from build123d import *

# Parameters (mm, degrees)
BOSS_EXTRUDE1_DEPTH = 6
SKETCH3_W           = 96
SKETCH3_H           = 45.5
BOSS_EXTRUDE2_DEPTH = 6
CUT_EXTRUDE1_DEPTH  = 6
CUT_EXTRUDE2_DEPTH  = 91.403621508
SKETCH9_W           = 27
SKETCH9_H           = 33.5
CUT_EXTRUDE3_DEPTH  = 91.403621508
CHAMFER1_SIZE       = 2
SKETCH11_R          = 2
CUT_EXTRUDE4_DEPTH  = 91.403621508
CUT_EXTRUDE6_START  = 0.01
SKETCH12_W          = 8
SKETCH12_H          = 6.6
CUT_EXTRUDE6_DEPTH  = 91.493120288


with BuildPart() as part:
    # Sketch2 → Boss-Extrude1 (new body)
    with BuildSketch(Plane(origin=(0, 0, 0), x_dir=(1, 0, 0), z_dir=(0, 1, 0))):
        with BuildLine():
            Line((27.190997647, 15.698729811), (53.17175976, 30.698729811))
            Line((53.17175976, 30.698729811), (48, 39.65648048))
            Line((48, 39.65648048), (48, 50))
            Line((48, 50), (-48, 50))
            Line((-48, 50), (-48, 39.65648048))
            Line((-48, 39.65648048), (-53.17175976, 30.698729811))
            Line((-53.17175976, 30.698729811), (-27.190997647, 15.698729811))
            ThreePointArc((-27.190997647, 15.698729811), (0, 31.397459622), (27.190997647, 15.698729811))
        make_face()
    extrude(amount=BOSS_EXTRUDE1_DEPTH)

    # Sketch3 → Boss-Extrude2 (add)
    with BuildSketch(Plane(origin=(0, -21.650635095, -37.5), x_dir=(-1, 0, 0), z_dir=(0, -0.500000000000001, -0.866025403784438))):
        with Locations((0, 47.75)):
            Rectangle(SKETCH3_W, SKETCH3_H)
    extrude(amount=-BOSS_EXTRUDE2_DEPTH)

    # Sketch4 → Cut-Extrude1 (cut)
    with BuildSketch(Plane(origin=(0, -21.650635095, -37.5), x_dir=(-1, 0, 0), z_dir=(0, -0.5000000000000009, -0.8660254037844383))):
        Polygon((24, 70.5), (24, 25), (24, 15), (-7, 15), (-7, 25), (-7, 70.5), align=None)
    extrude(amount=-CUT_EXTRUDE1_DEPTH, mode=Mode.SUBTRACT)

    # Sketch8 → Cut-Extrude2 (cut, through all)
    with BuildSketch(Plane(origin=(0, -21.650635095, -37.5), x_dir=(-1, 0, 0), z_dir=(0, -0.500000000000001, -0.8660254037844382))):
        Polygon((32, 64.5), (30, 62.5), (30, 33), (32, 31), (40, 31), (42, 33), (42, 62.5), (40, 64.5), align=None)
    extrude(amount=-CUT_EXTRUDE2_DEPTH, mode=Mode.SUBTRACT)

    # Sketch9 → Cut-Extrude3 (cut, through all)
    with BuildSketch(Plane(origin=(0, -21.650635095, -37.5), x_dir=(-1, 0, 0), z_dir=(0, -0.500000000000001, -0.8660254037844382))):
        with Locations((-28.5, 47.75)):
            Rectangle(SKETCH9_W, SKETCH9_H)
    extrude(amount=-CUT_EXTRUDE3_DEPTH, mode=Mode.SUBTRACT)

    # Chamfer1
    chamfer1_edges = [part.edges().sort_by_distance(p)[0] for p in [
        (15, 35.708003449, -67.151923789),
        (15, 6.696152423, -50.401923789),
        (42, 6.696152423, -50.401923789),
        (42, 35.708003449, -67.151923789),
    ]]
    chamfer(chamfer1_edges, length=CHAMFER1_SIZE)

    # Sketch11 → Cut-Extrude4 (cut, through all)
    with BuildSketch(Plane(origin=(0, -21.650635095, -37.5), x_dir=(-1, 0, 0), z_dir=(0, -0.500000000000001, -0.8660254037844382))):
        with Locations(Location((28, 66.5, 0), (0, 0, 90))):
            Circle(SKETCH11_R)
        with Locations(Location((44, 66.5, 0), (0, 0, 90))):
            Circle(SKETCH11_R)
        with Locations(Location((-11, 66.5, 0), (0, 0, 90))):
            Circle(SKETCH11_R)
        with Locations(Location((28, 29, 0), (0, 0, 90))):
            Circle(SKETCH11_R)
        with Locations(Location((44, 29, 0), (0, 0, 90))):
            Circle(SKETCH11_R)
        with Locations(Location((-11, 29, 0), (0, 0, 90))):
            Circle(SKETCH11_R)
    extrude(amount=-CUT_EXTRUDE4_DEPTH, mode=Mode.SUBTRACT)

    # Sketch12 → Cut-Extrude6 (cut, through all)
    with BuildSketch(Plane(origin=(0, -18.650635095, -32.303847577), x_dir=(1, 0, 0), z_dir=(0, 0.500000000000001, 0.8660254037844382)).offset(CUT_EXTRUDE6_START)):
        with Locations((11, 29)):
            Rectangle(SKETCH12_W, SKETCH12_H)
        with Locations((-28, 29)):
            Rectangle(SKETCH12_W, SKETCH12_H)
        with Locations((-44, 29)):
            Rectangle(SKETCH12_W, SKETCH12_H)
    extrude(amount=CUT_EXTRUDE6_DEPTH, mode=Mode.SUBTRACT)


solid = part.part
Can you work these out from the model? Positions are in its coordinate system, mm. A direction names the side the tool comes from. Round coordinates to 2 decimals unless told otherwise and drop trailing zeros. Order: outer loops, then holes, each group sorted by start corner. A loop starts at its lowest first (then second) coordinate and runs counter-clockwise, first axis right, second up. Notation, with made-up numbers: (88, 34) - (138, 34) arc R33 ccw to (138, 62) - close; hole circle Ø1 at (19.25, 31). An arc over 180 degrees is marked (long way). Answer in a Markdown table with one row per item.
(1) Which directions (+Z, -Z, +X, -X, +Y, -Y) give clear straight access to the entire face, cutting with the end or side of a thin tool? Please do faces 1 (the face through (-1, 6, -35)), 2 (the face through (-8.717, 3.042, -44.828)), 3 (the face through (10.944, 4.789, -43.105)).
From the geometry:
| item | result |
|---|---|
| face 1 | +Z, +X, -X, +Y |
| face 2 | -Z, -Y |
| face 3 | +Y |
(2) Suppose I cut it at A-A, the plane y = 18.5. Please give me the cut outline in (x, z).
From the geometry:
| item | result |
|---|---|
| outline | (-48, -60.68) - (-42, -60.68) - (-42, -53.75) - (-48, -53.75) - close; (-30, -60.68) - (-24, -60.68) - (-24, -53.75) - (-30, -53.75) - close; (7, -60.68) - (15, -60.68) - (15, -53.75) - (7, -53.75) - close; (42, -60.68) - (48, -60.68) - (48, -53.75) - (42, -53.75) - close |
(3) For P1, Ø4, axis at x = -34.5, y = 7.5, coming from the +Z side; P2, Ø0.7, axis at y = 4.5, z = -44.5, coming from the -X side; P3, Ø15, axis at y = 11.5, z = -53.5, coming from the +X side; P4, Ø12, axis at y = 35.5, z = -50.5, coming from the +X side, each with a flat end and sliding along its axis, tell me the tip position at first contact or that it passes through.
From the geometry:
| item | result |
|---|---|
| P1 | stops at z = -19.15 |
| P2 | stops at x = -40 |
| P3 | stops at x = 48 |
| P4 | passes through |
(4) Suppose I cut it at C-C, the plane x = 18.5. Please give me the cut outline in (y, z).
From the geometry:
| item | result |
|---|---|
| outline | (0, -50) - (5.2, -53) - (8.2, -47.8) - (6, -46.54) - (6, -25.37) - (0, -25.37) - close; (34.21, -69.75) - (39.4, -72.75) - (42.4, -67.55) - (37.21, -64.55) - close |
(5) Suppose I cut it at B-B, the plane z = -19.5. Please give me the cut outline in (x, y) (3 decimals).
From the geometry:
| item | result |
|---|---|
| outline | (-33.775, 0) - (-24.608, 0) - (-24.608, 6) - (-33.775, 6) - close; (24.608, 0) - (33.775, 0) - (33.775, 6) - (24.608, 6) - close |
(6) Please list where these lines run through material, in increasing order: L1, parallel to X at y = 8.5, z = -54; L2, parallel to Y at x = 22.5, z = -40; L3, parallel to X at y = 37.5, z = -66. Write a range as from..to.
From the geometry:
| item | result |
|---|---|
| L1 | x = -48..-42, -30..-24, 7..15, 42..48 |
| L2 | y = 0..6 |
| L3 | x = -48..-45.72, -42.28..-29.72, -26.28..-24, 7..9.28, 12.72..48 |
(7) If we mould it in two halves opening along Z, with no side actions, what happens to faces 4 (the face through (12.983, 37.194, -68.058)), 5 (the face through (-40.986, 7.529, -50.931)), 6 (the face through (48, 20, -56)), 7 (the face through (7, 5, -44))? For each: released by +Z, released by -Z, zero draft, split by the parting line, or undercut.
From the geometry:
| item | result |
|---|---|
| face 4 | undercut |
| face 5 | released by -Z |
| face 6 | zero draft |
| face 7 | undercut |
(8) Suppose I cut it at D-D, the plane z = -62. Please give me the cut outline in (x, y), plus the area to 3 significant figures.
From the geometry:
| item | result |
|---|---|
| outline | (-48, 20.78) - (-42, 20.78) - (-42, 32.78) - (-48, 32.78) - close; (-30, 20.78) - (-24, 20.78) - (-24, 32.78) - (-30, 32.78) - close; (7, 20.78) - (15, 20.78) - (15, 32.78) - (7, 32.78) - close; (42, 20.78) - (48, 20.78) - (48, 32.78) - (42, 32.78) - close |
| area | 312 mm2 |
